Geometry check sheet. Reference: the model listing, model coordinates, mm. Coordinates: 2 decimals unless noted, no trailing zeros. Write each loop counter-clockwise with the first axis right and the second up, starting at its lowest first coordinate (ties: lowest second). Pieces come first, ordered by that corner, then holes. Notation, with made-up numbers: (29, 0) -> (87, 0) arc R23 ccw to (87, 38) -> close; hole circle Ø11 at (2.5, -6). An arc over 180 degrees is marked (long way). Use a Markdown table: item, result.
```python
from build123d import *

# Parameters (mm, degrees)
SKETCH_1_R      = 2.5
EXTRUDE_1_DEPTH = 5
EXTRUDE_START   = 3
SKETCH_2_R      = 5
SKETCH_2_R_2    = 2.5
EXTRUDE_2_DEPTH = 3


with BuildPart() as part:
    # 草图1 → 凸台-拉伸1 (new body)
    with BuildSketch(Plane(origin=(0, 0, 0), x_dir=(1, 0, 0), z_dir=(0, 1, 0))):
        with BuildLine():
            Line((-34.30294509, -6.015613436), (0.69705491, -6.015613436))
            ThreePointArc((0.69705491, -6.015613436), (5.69705491, -11.015613436), (0.69705491, -16.015613436))
            Line((0.69705491, -16.015613436), (-34.30294509, -16.015613436))
            ThreePointArc((-34.30294509, -16.015613436), (-39.30294509, -11.015613436), (-34.30294509, -6.015613436))
        make_face()
        with Locations(Location((-34.30294509, -11.015613436, 0), (0, 0, 270))):
            Circle(SKETCH_1_R, mode=Mode.SUBTRACT)
    extrude(amount=EXTRUDE_1_DEPTH)

    # 草图2 → 凸台-拉伸2 (add)
    with BuildSketch(Plane.XZ.offset(EXTRUDE_START)):
        with Locations(Location((-34.30294509, 11.015613436, 0), (0, 0, 270))):
            Circle(SKETCH_2_R)
        with Locations(Location((-34.30294509, 11.015613436, 0), (0, 0, 270))):
            Circle(SKETCH_2_R_2, mode=Mode.SUBTRACT)
    extrude(amount=-EXTRUDE_2_DEPTH)


solid = part.part
```
Item 1: Thickness scan on L1, parallel to Y at x = 2, z = 11; L2, parallel to X at y = 4.5, z = 12; L3, parallel to X at y = 3.5, z = 10.5. Record the ranges inside material, lowest first. Write a range as [from, to].
Answer block:
| item | result |
|---|---|
| L1 | y = [0, 5] |
| L2 | x = [-39.21, -36.6], [-32, 5.6] |
| L3 | x = [-39.28, -36.75], [-31.86, 5.67] |
Item 2: Section check B-B on y = 2.5. Record the boundary of the cut face in (x, z), then the cut area to 3 significant figures.
Answer block:
| item | result |
|---|---|
| outline | (-34.3, 6.02) -> (0.7, 6.02) arc R5 ccw to (0.7, 16.02) -> (-34.3, 16.02) arc R5 ccw to start; hole circle Ø5 at (-34.3, 11.02) |
| area | 409 mm^2 |
Item 3: Section check C-C on x = -17. Record the boundary of the cut face in (y, z), then the cut area to 3 significant figures.
Answer block:
| item | result |
|---|---|
| outline | (0, 6.02) -> (5, 6.02) -> (5, 16.02) -> (0, 16.02) -> close |
| area | 50.0 mm^2 |
Item 4: Section check A-A on z = 9. Record the boundary of the cut face in (x, y).
Answer block:
| item | result |
|---|---|
| outline | (-38.88, -3) -> (-35.78, -3) -> (-35.78, 5) -> (-38.88, 5) -> close; (-32.82, -3) -> (-29.73, -3) -> (-29.73, 0) -> (5.27, 0) -> (5.27, 5) -> (-32.82, 5) -> close |
Item 5: Depth check by flat-ended pin: P1, Ø3, axis at x = -18, z = 11, coming from the -Y side; P2, Ø3, axis at y = 2.5, z = 15, coming from the +X side; P3, Ø4.5, axis at x = -34.3, z = 11.02, coming from the +Y side; P4, Ø3, axis at y = 2.5, z = 8.5, coming from the -X side. Enter the tip coordinate at first touch or a pass-through.
Answer block:
| item | result |
|---|---|
| P1 | stops at y = 0 |
| P2 | stops at x = 5.04 |
| P3 | passes through |
| P4 | stops at x = -39.2 |
Item 6: Section check D-D on z = 11.75. Record the boundary of the cut face in (x, y), then the cut area to 3 significant figures.
Answer block:
| item | result |
|---|---|
| outline | (-39.25, -3) -> (-36.69, -3) -> (-36.69, 5) -> (-39.25, 5) -> close; (-31.91, -3) -> (-29.36, -3) -> (-29.36, 0) -> (5.64, 0) -> (5.64, 5) -> (-31.91, 5) -> close |
| area | 216 mm^2 |
